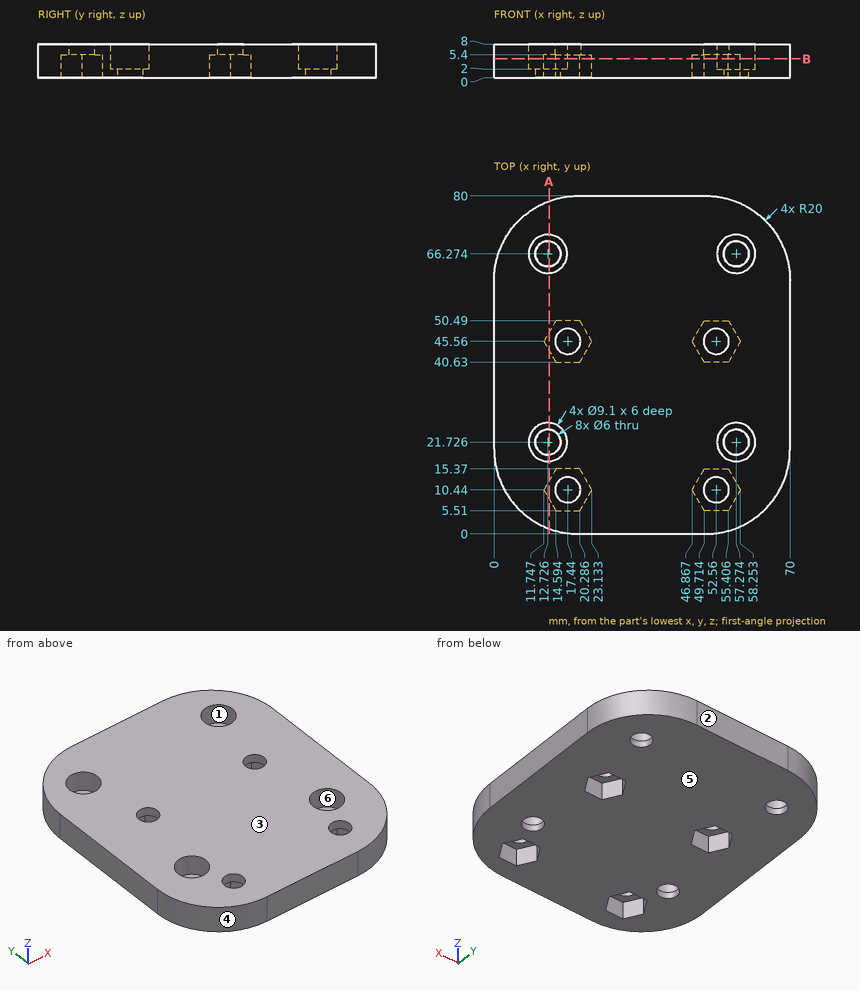
Print and shaded views of the part. All mm, measured from the part's lowest x, y and z. A direction names the side the tool comes from. Give positions to 0.01 mm unless a question says otherwise; leave off trailing zeros. Loops run counter-clockwise (first coordinate to the right, second up) from the corner with the lowest first, then second, coordinate; pieces in that order, holes last. Notation, with made-up numbers: (29.25, 65.25) - (56.25, 65.25) arc R32 ccw to (56.25, 102.25) - close; hole circle Ø9 at (38.5, 15). An arc over 180 degrees is marked (long way). One line per item, written item: value. Start each with the question number.
1. Slice it at A-A (x = 13). List the corners of the cut face in (y, z) (1 decimal), plus the area to 3 significant figures.
2. Probe L1, parallel to Y at x = 19.5, z = 1.5; L2, parallel to X at y = 67.5, z = 3 (1 decimal); L3, parallel to Y at x = 56.5, z = 7.5 (1 decimal). List the from-to ranges inside material, lowest first. Write a range as from..to.
3. Pin check, flat tips, straight feed: pin 1 (2.5 mm diameter, centred on x = 53.5, z = 4, fed in from -Y); pin 2 (3 mm diameter, centred on x = 15.5, y = 47, fed in from -Z); pin 3 (8 mm diameter, centred on x = 12.73, y = 21.73, fed in from +Z); pin 4 (5.5 mm diameter, centred on x = 52.56, y = 10.44, fed in from +Z). Stop position of each tip, or through.
4. Which spindle directions (+Z, -Z, +X, -X, +Y, -Y) get a long thin tool onto all of the face, cutting with end or side? Do the marked faces 5 and 6. Say none if no direction does.
5. Slice it at B-B (z = 4.5). Give the number of separate pieces and of enclosed holes in the cut face, plus the area to 3 significant figures.
6. Pull direction Y, two halves, no side cores. Call the marked faces 1, 2, 3 and 4: pulls with the +Y half, pulls with the -Y half, needs draft (parallel to the pull), parting line crosses it, or undercut.
Solution:
1. outline: (1.3, 0) - (8.3, 0) - (8.3, 5.4) - (12.6, 5.4) - (12.6, 0) - (18.7, 0) - (18.7, 2) - (17.2, 2) - (17.2, 8) - (1.3, 8) - close; (24.7, 0) - (43.4, 0) - (43.4, 5.4) - (47.7, 5.4) - (47.7, 0) - (63.3, 0) - (63.3, 2) - (61.7, 2) - (61.7, 8) - (26.3, 8) - (26.3, 2) - (24.7, 2) - close; (69.3, 0) - (78.7, 0) - (78.7, 8) - (70.8, 8) - (70.8, 2) - (69.3, 2) - close
1. area: 440 mm^2
2. L1: y = 0.01..5.51, 15.37..40.63, 50.49..79.99
2. L2: x = 1.5..8.3, 17.1..52.9, 61.7..68.5
2. L3: y = 1.1..17.2, 26.2..61.8, 70.8..78.9
3. pin 1: stops at y = 0.13
3. pin 2: stops at z = 5.4
3. pin 3: stops at z = 2
3. pin 4: passes through
4. face 5: -Z, +X, -X, +Y, -Y
4. face 6: +Z
5. separate pieces: 1
5. enclosed holes: 8
5. area: 4,660 mm^2
6. face 1: undercut
6. face 2: pulls with the +Y half
6. face 3: needs draft
6. face 4: pulls with the -Y half
